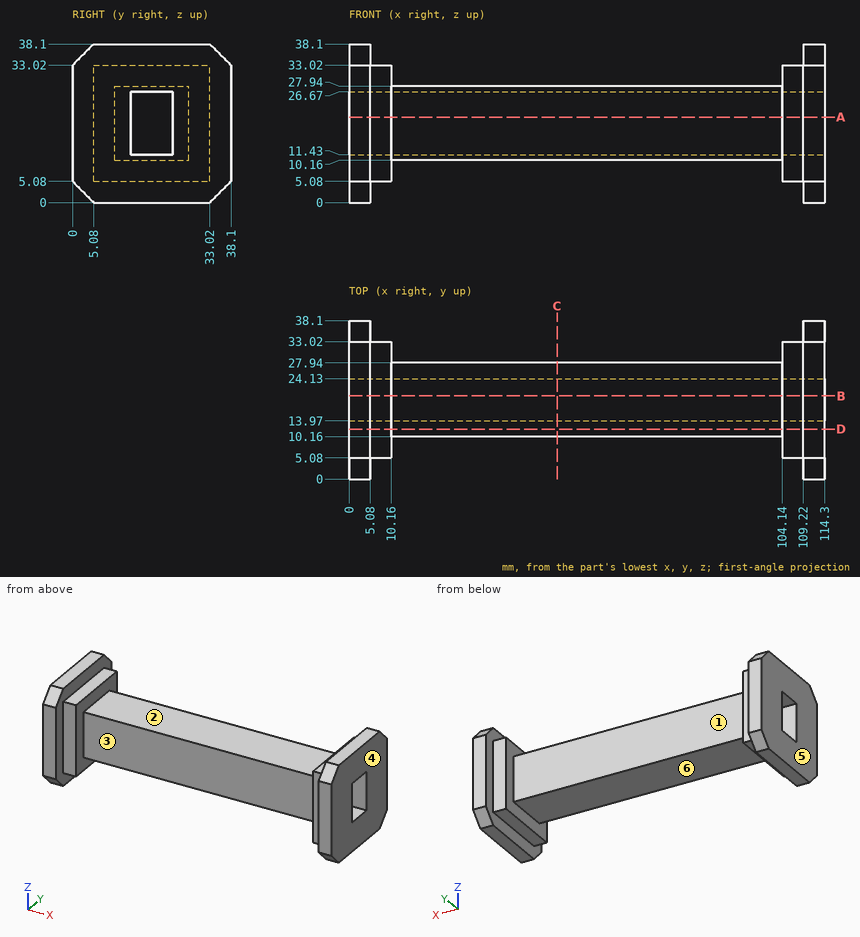
Source: three-view drawing plus pictorial views. Frame: mm from the lowest corner of the part. A direction names the side the tool comes from. Give positions to 0.01 mm unless a question says otherwise; leave off trailing zeros. Loops run counter-clockwise (first coordinate to the right, second up) from the corner with the lowest first, then second, coordinate; pieces in that order, holes last. Notation, with made-up numbers: (53.25, 8.25) -> (71.25, 8.25) arc R6 ccw to (71.25, 17.25) -> close; hole circle Ø6 at (18, 12). An arc over 180 degrees is marked (long way). Use a Markdown table: item, result. Add a question column.
(1) First-contact query: pin 1 Ø14 at (x, y) = (79.5, 18) entering from -Z; pin 2 Ø4.5 at (x, z) = (83.5, 19) entering from +Y; pin 3 Ø2.5 at (x, y) = (105.5, 21) entering from +Z; pin 4 Ø2 at (y, z) = (16.5, 18.5) entering from -X. Flat tips, straight axial feed; report the tip coordinate or a pass-through.
(2) Section query C-C (x = 50). Output: boundary loops of the cut face in (y, z), then the cut area to 3 significant figures.
(3) Section query A-A (z = 20.5). Output: boundary loops of the cut face in (x, y), then the cut area to 3 significant figures.
(4) Section query B-B (y = 20). Output: boundary loops of the cut face in (x, z).
(5) Section query D-D (y = 12). Output: boundary loops of the cut face in (x, z).
(6) Pull-direction query (X, two-part tool) for the marked faces 4, 5 and 6; classes: +X half, -X half, draft (parallel to the pull), parting line (faces both ways), or undercut.
(7) Ray query, line 1 (Y direction, x = 72, z = 21); line 2 (Z direction, x = 73, y = 23); line 3 (X direction, y = 17, z = 30). Return the intervals inside material, ascending.
(8) Access query for the marked faces 1, 2 and 3. Directions: +Z, -Z, +X, -X, +Y, -Y. A direction counts if a zero-diameter tool reaches every point of the face in a straight line with its end or side. Return the directions, or none.
Checked values:
| question | item | result |
|---|---|---|
| 1 | pin 1 | z = 10.16 |
| 1 | pin 2 | y = 27.94 |
| 1 | pin 3 | z = 33.02 |
| 1 | pin 4 | through |
| 2 | outline | (10.16, 10.16) -> (27.94, 10.16) -> (27.94, 27.94) -> (10.16, 27.94) -> close; hole (13.97, 11.43) -> (24.13, 11.43) -> (24.13, 26.67) -> (13.97, 26.67) -> close |
| 2 | area | 161 mm^2 |
| 3 | outline | (0, 0) -> (5.08, 0) -> (5.08, 5.08) -> (10.16, 5.08) -> (10.16, 10.16) -> (104.14, 10.16) -> (104.14, 5.08) -> (109.22, 5.08) -> (109.22, 0) -> (114.3, 0) -> (114.3, 13.97) -> (0, 13.97) -> close; (0, 24.13) -> (114.3, 24.13) -> (114.3, 38.1) -> (109.22, 38.1) -> (109.22, 33.02) -> (104.14, 33.02) -> (104.14, 27.94) -> (10.16, 27.94) -> (10.16, 33.02) -> (5.08, 33.02) -> (5.08, 38.1) -> (0, 38.1) -> close |
| 3 | area | 1,180 mm^2 |
| 4 | outline | (0, 0) -> (5.08, 0) -> (5.08, 5.08) -> (10.16, 5.08) -> (10.16, 10.16) -> (104.14, 10.16) -> (104.14, 5.08) -> (109.22, 5.08) -> (109.22, 0) -> (114.3, 0) -> (114.3, 11.43) -> (0, 11.43) -> close; (0, 26.67) -> (114.3, 26.67) -> (114.3, 38.1) -> (109.22, 38.1) -> (109.22, 33.02) -> (104.14, 33.02) -> (104.14, 27.94) -> (10.16, 27.94) -> (10.16, 33.02) -> (5.08, 33.02) -> (5.08, 38.1) -> (0, 38.1) -> close |
| 5 | outline | (0, 0) -> (5.08, 0) -> (5.08, 5.08) -> (10.16, 5.08) -> (10.16, 10.16) -> (104.14, 10.16) -> (104.14, 5.08) -> (109.22, 5.08) -> (109.22, 0) -> (114.3, 0) -> (114.3, 38.1) -> (109.22, 38.1) -> (109.22, 33.02) -> (104.14, 33.02) -> (104.14, 27.94) -> (10.16, 27.94) -> (10.16, 33.02) -> (5.08, 33.02) -> (5.08, 38.1) -> (0, 38.1) -> close |
| 6 | face 4 | +X half |
| 6 | face 5 | -X half |
| 6 | face 6 | undercut |
| 7 | line 1 | 10.16 to 13.97, 24.13 to 27.94 |
| 7 | line 2 | 10.16 to 11.43, 26.67 to 27.94 |
| 7 | line 3 | 0 to 10.16, 104.14 to 114.3 |
| 8 | face 1 | +Z, -Z, +Y |
| 8 | face 2 | +Z, +Y, -Y |
| 8 | face 3 | +Z, -Z, -Y |
